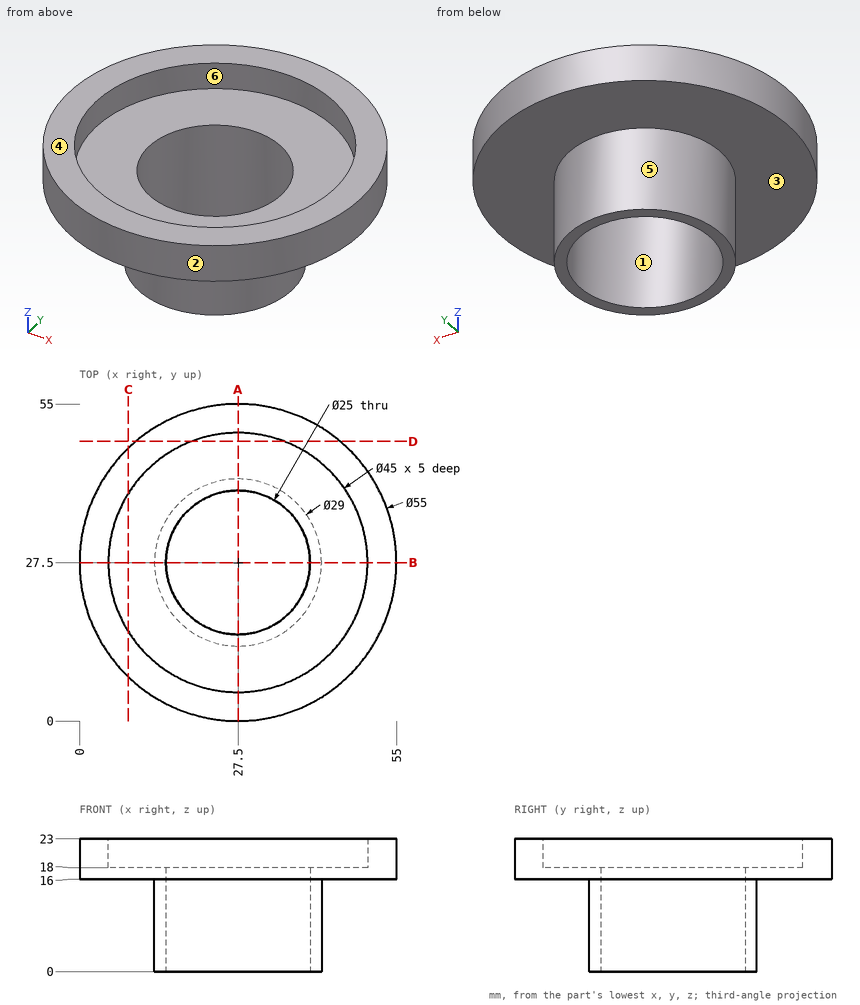
Drawing for the job (mm, zero at the part's lowest x, y, z). A direction names the side the tool comes from. Coordinates: 2 decimals unless noted, no trailing zeros. Order: outer loops, then holes, each group sorted by start corner. A loop starts at its lowest first (then second) coordinate and runs counter-clockwise, first axis right, second up.
Item 1: Band-saw the part on C-C on x = 8.5. List the corners of the cut face in (y, z), plus the area to 3 significant figures.
Check sheet entries:
outline: (7.62, 16) - (47.38, 16) - (47.38, 23) - (39.55, 23) - (39.55, 18) - (15.45, 18) - (15.45, 23) - (7.62, 23) - close
area: 158 mm2
Item 2: Pin check, flat tips, straight feed: pin 1 Ø5 at (x, y) = (38, 7) entering from -Z; pin 2 Ø20 at (x, y) = (27.5, 27.5) entering from -Z; pin 3 Ø2 at (y, z) = (10, 17.5) entering from +X; pin 4 Ø3 at (y, z) = (23, 18.5) entering from +X. Stop position of each tip, or through.
Check sheet entries:
pin 1: stops at z = 16
pin 2: passes through
pin 3: stops at x = 49.5
pin 4: stops at x = 54.84
Item 3: Two-plate mould, pull along X, no slides. Class the marked faces 1, 2 and 3: +X half, -X half, draft (parallel to the pull), parting line (faces both ways), or undercut.
Check sheet entries:
face 1: undercut
face 2: parting line
face 3: draft
Item 4: 3-axis set-ups, long thin cutter, end or side, ignore diameter. For the marked faces 4, 5 and 6: which of +Z, -Z, +X, -X, +Y, -Y reach the whole face in a straight line?
Check sheet entries:
face 4: +Z, +X, -X, +Y, -Y
face 5: -Z
face 6: +Z
Item 5: Band-saw the part on A-A on x = 27.5. List the corners of the cut face in (y, z), plus the area to 3 significant figures.
Check sheet entries:
outline: (0, 16) - (13, 16) - (13, 0) - (15, 0) - (15, 18) - (5, 18) - (5, 23) - (0, 23) - close; (40, 0) - (42, 0) - (42, 16) - (55, 16) - (55, 23) - (50, 23) - (50, 18) - (40, 18) - close
area: 174 mm2
Item 6: Drill centre lines: L1, parallel to Y at x = 27.5, z = 21.05; L2, parallel to Y at x = 27.5, z = 5; L3, parallel to Z at x = 39, y = 16. Where is each one in solid material? Low to high.
Check sheet entries:
L1: y = 0 to 5, 50 to 55
L2: y = 13 to 15, 40 to 42
L3: z = 16 to 18
Item 7: Band-saw the part on D-D on y = 48.5. List the corners of the cut face in (x, z).
Check sheet entries:
outline: (9.74, 16) - (45.26, 16) - (45.26, 23) - (35.58, 23) - (35.58, 18) - (19.42, 18) - (19.42, 23) - (9.74, 23) - close
